from build123d import *

# Parameters (mm, degrees)
SKETCH1_R           = 27.94
BOSS_EXTRUDE1_DEPTH = 3.048
SKETCH2_R           = 26.416
BOSS_EXTRUDE2_DEPTH = 105.156
SKETCH3_R           = 27.686
BOSS_EXTRUDE3_DEPTH = 3.048
SKETCH4_R           = 26.162
CUT_EXTRUDE1_DEPTH  = 4.064
SKETCH5_R           = 22.733
BOSS_EXTRUDE4_DEPTH = 8.382
SKETCH6_R           = 16.256
BOSS_EXTRUDE5_DEPTH = 3.556
SKETCH7_R           = 11.303
BOSS_EXTRUDE6_DEPTH = 2.794
SKETCH8_R           = 8.128
BOSS_EXTRUDE7_DEPTH = 13.208
FILLET1_R           = 7.62
FILLET2_R           = 1.27


with BuildPart() as part:
    # Sketch1 → Boss-Extrude1 (new body)
    with BuildSketch(Plane(origin=(0, 0, 0), x_dir=(1, 0, 0), z_dir=(0, 1, 0))):
        with Locations(Location((0, 0, 0), (0, 0, 90))):
            Circle(SKETCH1_R)
    extrude(amount=BOSS_EXTRUDE1_DEPTH)

    # Sketch2 → Boss-Extrude2 (add)
    with BuildSketch(Plane(origin=(0, 3.048, 0), x_dir=(1, 0, 0), z_dir=(0, 1, 0))):
        with Locations(Location((0, 0, 0), (0, 0, 270))):
            Circle(SKETCH2_R)
    extrude(amount=BOSS_EXTRUDE2_DEPTH)

    # Sketch3 → Boss-Extrude3 (add)
    with BuildSketch(Plane(origin=(0, 108.204, 0), x_dir=(1, 0, 0), z_dir=(0, 1, 0))):
        with Locations(Location((0, 0, 0), (0, 0, 90))):
            Circle(SKETCH3_R)
    extrude(amount=BOSS_EXTRUDE3_DEPTH)

    # Sketch4 → Cut-Extrude1 (cut)
    with BuildSketch(Plane(origin=(0, 111.252, 0), x_dir=(1, 0, 0), z_dir=(0, 1, 0))):
        with Locations(Location((0, 0, 0), (0, 0, 270))):
            Circle(SKETCH4_R)
    extrude(amount=-CUT_EXTRUDE1_DEPTH, mode=Mode.SUBTRACT)

    # Sketch5 → Boss-Extrude4 (add)
    with BuildSketch(Plane(origin=(0, 107.188, 0), x_dir=(1, 0, 0), z_dir=(0, 1, 0))):
        with Locations(Location((0, 0, 0), (0, 0, 270))):
            Circle(SKETCH5_R)
    extrude(amount=BOSS_EXTRUDE4_DEPTH)

    # Sketch6 → Boss-Extrude5 (add)
    with BuildSketch(Plane(origin=(0, 115.57, 0), x_dir=(1, 0, 0), z_dir=(0, 1, 0))):
        with Locations(Location((0, 0, 0), (0, 0, 270))):
            Circle(SKETCH6_R)
    extrude(amount=BOSS_EXTRUDE5_DEPTH)

    # Sketch7 → Boss-Extrude6 (add)
    with BuildSketch(Plane(origin=(0, 119.126, 0), x_dir=(1, 0, 0), z_dir=(0, 1, 0))):
        with Locations(Location((0, 0, 0), (0, 0, 270))):
            Circle(SKETCH7_R)
    extrude(amount=BOSS_EXTRUDE6_DEPTH)

    # Sketch8 → Boss-Extrude7 (add)
    with BuildSketch(Plane(origin=(0, 121.92, 0), x_dir=(1, 0, 0), z_dir=(0, 1, 0))):
        with Locations(Location((0, 0, 0), (0, 0, 90))):
            Circle(SKETCH8_R)
    extrude(amount=BOSS_EXTRUDE7_DEPTH)

    # Fillet1
    # the kernel refuses this fillet: 7.62 mm, written as the material it takes off along each edge
    with BuildSketch(Plane(origin=(0, 115.57, 0), x_dir=(0, 0, 1), z_dir=(-1, 0, 0))) as fillet1_piece_1:
        with BuildLine():
            CenterArc((15.113, -7.533787295), FILLET1_R, 0, 81.373073441)
            Line((16.256, 0), (16.27886, 0.150675746))
            ThreePointArc((16.27886, 0.150675746), (19.4945, 0.1524), (22.733, 0.1524))
            Line((22.733, 0.1524), (22.8854, 0))
            Line((22.8854, 0), (22.8854, -7.533787295))
            Line((22.8854, -7.533787295), (22.733, -7.533787295))
        make_face()
    revolve(axis=Axis((0, 115.57, 0), (0, 1, 0)), mode=Mode.SUBTRACT)

    # Fillet2
    fillet2_edges = [part.edges().sort_by_distance(p)[0] for p in [
        (0, 119.126, -16.256),
    ]]
    fillet(fillet2_edges, radius=FILLET2_R)


solid = part.part
Check sheet for the modelled part. Datum: model origin and axes. Units: mm. A direction names the side the tool comes from. Give positions to 0.01 mm unless a question says otherwise; leave off trailing zeros. Write each loop counter-clockwise with the first axis right and the second up, starting at its lowest first coordinate (ties: lowest second). Pieces come first, ordered by that corner, then holes. Notation, with made-up numbers: (-3.75, -12) -> (12.25, -12) arc R25 ccw to (12.25, 24) -> close; hole circle Ø10 at (-22.75, 11). An arc over 180 degrees is marked (long way). Use one line per item in the form item = value. Start each with the question number.
1. Go/stop test with flat-tipped pins: P1, Ø10, axis at y = 100.5, z = -16.5, coming from the -X side; P2, Ø8, axis at y = 101.5, z = 6, coming from the -X side; P3, Ø6, axis at x = -3, z = 21, coming from the +Y side. Record where each tip stops, or that it passes through.
2. Section check C-C (y = 74). Record the cut outline in (x, z), and give its area (3 significant figures).
3. Section check D-D (x = 24). Record the cut outline in (y, z), and give its area (3 significant figures).
4. Access from +Z, -Z, +X, -X, +Y, -Y to the whole of each face (thin tool, end or side, straight path). Record for faces 1 (the cylindrical face through (7.935, 54.89, 25.196)), 2 (the flat face through (0, 135.128, 0)), 3 (the cylindrical face through (22.54, 107.61, -2.96)).
5. Mould release check, pull along Z, two halves, no side actions. Record for faces 4 (the cylindrical face through (-25.54, 109.25, -5.67)), 5 (the flat face through (27, 108.204, 0)), 6 (the cylindrical face through (-27.7, 1.5, 3.64)): pulls with the +Z half, pulls with the -Z half, needs draft (parallel to the pull), parting line crosses it, or undercut.
6. Thickness scan on line 1 along X through (y, z) = (108.35, 0); line 2 along Y through (x, z) = (22.5, -8); line 3 along X through (y, z) = (109.15, 0). Record the ranges inside material, lowest first. Write a range as from..to.
Conclusion:
q1.P1 = -23.78
q1.P2 = -26.34
q1.P3 = 115
q2.outline = circle Ø52.83 at (0, 0)
q2.area = 2,190 mm²
q3.outline = (0, -14.31) -> (3.05, -14.31) -> (3.05, -11.04) -> (108.2, -11.04) -> (108.2, -13.8) -> (111.25, -13.8) -> (111.25, -10.41) -> (107.19, -10.41) -> (107.19, 10.41) -> (111.25, 10.41) -> (111.25, 13.8) -> (108.2, 13.8) -> (108.2, 11.04) -> (3.05, 11.04) -> (3.05, 14.31) -> (0, 14.31) -> close
q3.area = 2,410 mm²
q4.face_1 = none
q4.face_2 = +Z, -Z, +X, -X, +Y
q4.face_3 = +Y
q5.face_4 = undercut
q5.face_5 = needs draft
q5.face_6 = parting line crosses it
q6.line_1 = -27.69..-26.16, -22.73..22.73, 26.16..27.69
q6.line_2 = 0..107.19
q6.line_3 = -27.69..-26.16, -22.65..22.65, 26.16..27.69
